For this review, take the finished solid that the model builds, in its own axes (mm). Face numbers are marked on the shaded views. A direction names the side the tool comes from. Round coordinates to 2 decimals unless told otherwise and drop trailing zeros. Order: outer loops, then holes, each group sorted by start corner. A loop starts at its lowest first (then second) coordinate and runs counter-clockwise, first axis right, second up. Notation, with made-up numbers: M 14.5,7.25 L 48.5,7.25 A19 cw 48.5,34.25 Z; hole C -2,-21.75 d2. An arc over 180 degrees is marked long. Answer in a Markdown table with one row per item. Add a question column.
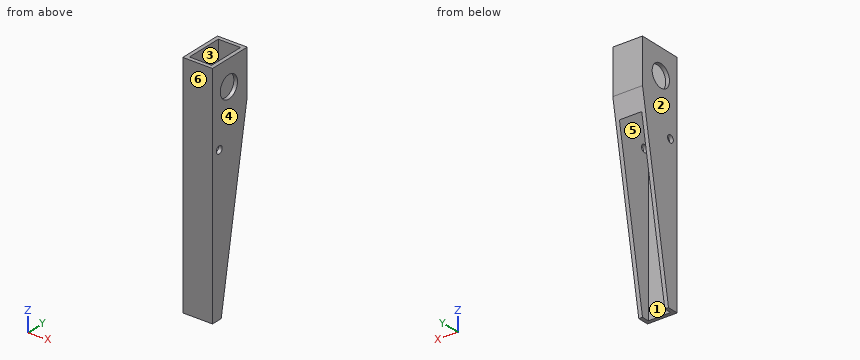
```python
from build123d import *

# Parameters (mm, degrees)
SKETCH1_W           = 3.175
SKETCH1_H           = 38.1
SKETCH1_W_2         = 19.05
SKETCH1_H_2         = 3.175
BOSS_EXTRUDE1_DEPTH = 196.5706
SKETCH2_R           = 9.5123
SKETCH2_R_2         = 3.175
SIDE_CUT_DEPTH      = 26.4


with BuildPart() as part:
    # Sketch1 → Boss-Extrude1 (new body)
    with BuildSketch(Plane.XY):
        with Locations((1.5875, 19.05)):
            Rectangle(SKETCH1_W, SKETCH1_H)
        with Locations((12.7, 1.5875)):
            Rectangle(SKETCH1_W_2, SKETCH1_H_2)
        Polygon((22.225, 3.175), (22.225, 0), (25.4, 0), (25.4, 38.1), (22.225, 38.1), (22.225, 34.925), align=None)
        with Locations((12.7, 36.5125)):
            Rectangle(SKETCH1_W_2, SKETCH1_H_2)
    extrude(amount=BOSS_EXTRUDE1_DEPTH)

    # Sketch2 → Side cut (cut, through all)
    with BuildSketch(Plane(origin=(25.4, 0, 0), x_dir=(0, 0, -1), z_dir=(1, 0, 0))):
        with Locations((-174.7266, 17.991529913)):
            Circle(SKETCH2_R)
        with Locations((-130.736416842, 7.4258361)):
            Circle(SKETCH2_R_2)
        Polygon((-158.4706, 38.1), (0, 9.525), (0, 38.1), align=None)
    extrude(amount=-SIDE_CUT_DEPTH, mode=Mode.SUBTRACT)


solid = part.part
```
1. Consider section A-A on x = 19.5. Write out the cut boundary in (y, z) (3 decimals), plus the area to 3 significant figures.
2. Clearance check with a flat-ended pin moving along its axis: pin 1 Ø3 at (x, z) = (20, 39) entering from +Y (3 decimals). State where the tip first meets the part, or that it passes through.
3. To check wall thickness, follow probe 1 along X at (y, z) = (10, 85.5) (3 decimals); probe 2 along Y at (x, z) = (6.75, 171) (3 decimals); probe 3 along Y at (x, z) = (20.5, 145.5) (3 decimals). State the ranges of each line that lie inside material, in increasing order. Write a range as [from, to].
4. Consider section D-D on y = 29.5. Write out the cut boundary in (x, z) (3 decimals), plus the area to 3 significant figures.
5. Consider section B-B on y = 20. Write out the cut boundary in (x, z) (3 decimals).
6. The part is to be moulded in two halves that separate along X. For the marked faces 3, 4, 5 and 6, say which applies: pulls with the +X half, pulls with the -X half, needs draft (parallel to the pull), parting line crosses it, or undercut.
7. For the marked faces 1 and 2, list the 3-axis set-ups (+Z, -Z, +X, -X, +Y, -Y) from which the entire face can be reached by the end or side of a thin tool; tool diameter is ignored.
8. Consider section C-C on z = 136. Write out the cut boundary in (x, y) (3 decimals), plus the area to 3 significant figures.
Solved:
| question | item | result |
|---|---|---|
| 1 | outline | M 0,0 L 3.175,0 L 3.175,196.571 L 0,196.571 Z; M 34.925,140.863 L 38.1,158.471 L 38.1,196.571 L 34.925,196.571 Z |
| 1 | area | 773 mm^2 |
| 2 | pin 1 | stops at y = 3.175 |
| 3 | probe 1 | x = [0, 3.175], [22.225, 25.4] |
| 3 | probe 2 | y = [0, 3.175], [34.925, 38.1] |
| 3 | probe 3 | y = [0, 3.175], [34.925, 35.761] |
| 4 | outline | M 0,110.777 L 3.175,110.777 L 3.175,196.571 L 0,196.571 Z; M 22.225,110.777 L 25.4,110.777 L 25.4,196.571 L 22.225,196.571 Z |
| 4 | area | 545 mm^2 |
| 5 | outline | M 0,58.092 L 3.175,58.092 L 3.175,165.429 L 0,165.429 Z; M 0,184.024 L 3.175,184.024 L 3.175,196.571 L 0,196.571 Z; M 22.225,58.092 L 25.4,58.092 L 25.4,165.429 L 22.225,165.429 Z; M 22.225,184.024 L 25.4,184.024 L 25.4,196.571 L 22.225,196.571 Z |
| 6 | face 3 | undercut |
| 6 | face 4 | pulls with the +X half |
| 6 | face 5 | undercut |
| 6 | face 6 | needs draft |
| 7 | face 1 | +Z, -Z |
| 7 | face 2 | +Z, -Z, -X, +Y, -Y |
| 8 | outline | M 0,0 L 25.4,0 L 25.4,34.048 L 22.225,34.048 L 22.225,3.175 L 3.175,3.175 L 3.175,34.048 L 0,34.048 Z |
| 8 | area | 277 mm^2 |
